Here's how the part is built. I have some questions about the finished solid (model axes, mm). A direction names the side the tool comes from. Give positions to 0.01 mm unless a question says otherwise; leave off trailing zeros. Loops run counter-clockwise (first coordinate to the right, second up) from the corner with the lowest first, then second, coordinate; pieces in that order, holes last. Notation, with made-up numbers: (24.25, 79) - (56.25, 79) arc R12 cw to (56.25, 98) - close; hole circle Ø2 at (12.5, 84.5). An arc over 180 degrees is marked (long way). Use a Markdown table: item, result.
Autodesk Inventor part; units mm, degrees
ref_plane "r_pin_XY" through (0, 0, 0) normal (0, 1, 0) x (1, 0, 0)
ref_plane "r_pin_YZ" through (0, 0, 0) normal (1, 0, 0) x (0, 0, -1)
ref_plane "r_pin_ZX" through (0, 0, 0) normal (0, 0, -1) x (0, 1, 0)
sketch "Sketch_1" plane through (0, 0, 0) normal (0, 0, 1) x (1, 0, 0)
  line L0 (0, -20.5) -> (0, 20.5)
  line L1 (0, 20.5) -> (4.6, 20.5)
  line L2 (4.6, 20.5) -> (4.6, -20.5)
  line L3 (4.6, -20.5) -> (0, -20.5)
  line L4 (0, -20.5) -> (0, 20.5)
revolve "Revolution1" add sketch "Sketch_1" angle 360 about axis through (0, -20.5, 0) along (0, -1, 0)
sketch "Sketch_2" plane through (0, 0, -4.6) normal (0, 0, 1) x (1, 0, 0)
  line L0 (0, 20.5) -> (0, -20.5)
  line L1 (0, -20.5) -> (10.5, -20.5)
  arc A0 (10.5, -20.5) -> (18, -13) centre (10.5, -13) ccw
  line L2 (18, -13) -> (18, 13)
  arc A1 (18, 13) -> (10.5, 20.5) centre (10.5, 13) ccw
  line L3 (10.5, 20.5) -> (0, 20.5)
extrude "Extrusion1" add sketch "Sketch_2" along normal blind 2
sketch "Sketch_3" plane through (0, 0, 0) normal (0, 0, 1) x (1, 0, 0)
  line L0 (-41, 41) -> (-41, -41)
  line L1 (-41, -41) -> (41, -41)
  line L2 (41, -41) -> (41, 41)
  line L3 (41, 41) -> (-41, 41)
  line L4 (-4.6, 20.5) -> (-4.6, 10.35)
  line L5 (-4.6, 10.35) -> (4.85, 10.35)
  line L6 (4.85, 10.35) -> (4.85, -0.2)
  line L7 (4.85, -0.2) -> (-4.6, -0.2)
  line L8 (-4.6, -0.2) -> (-4.6, -10.05)
  line L9 (-4.6, -10.05) -> (4.85, -10.05)
  line L10 (4.85, -10.05) -> (4.85, -20.5)
  line L11 (4.85, -20.5) -> (18, -20.5)
  line L12 (18, -20.5) -> (18, 20.5)
  line L13 (18, 20.5) -> (-4.6, 20.5)
extrude "Extrusion2" cut sketch "Sketch_3" along normal mid plane 82
sketch "Sketch_4" plane through (0, 0, 0) normal (0, 0, 1) x (1, 0, 0)
  line L0 (0, -20.5) -> (0, 20.5)
  line L1 (0, 20.5) -> (2.5, 20.5)
  line L2 (2.5, 20.5) -> (2.5, -20.5)
  line L3 (2.5, -20.5) -> (0, -20.5)
  line L4 (0, -20.5) -> (0, 20.5)
revolve "Revolution2" cut sketch "Sketch_4" angle 360 about axis through (0, -20.5, 0) along (0, -1, 0)
sketch "Sketch_5" plane through (0, 12.5, 0) normal (0, 1, 0) x (1, 0, 0)
  line L0 (10.5, 2.6) -> (10.5, 4.6)
  line L1 (10.5, 4.6) -> (13.25, 4.6)
  line L2 (13.25, 4.6) -> (13.25, 2.6)
  line L3 (13.25, 2.6) -> (10.5, 2.6)
  line L4 (10.5, 2.6) -> (10.5, 4.6)
revolve "Revolution3" cut sketch "Sketch_5" angle 360 about axis through (10.5, 12.5, -2.6) along (0, 0, 1)
sketch "Sketch_7" plane through (0, -12.5, 0) normal (0, 1, 0) x (1, 0, 0)
  line L0 (10.5, 2.6) -> (10.5, 4.6)
  line L1 (10.5, 4.6) -> (13.25, 4.6)
  line L2 (13.25, 4.6) -> (13.25, 2.6)
  line L3 (13.25, 2.6) -> (10.5, 2.6)
  line L4 (10.5, 2.6) -> (10.5, 4.6)
revolve "Revolution4" cut sketch "Sketch_7" angle 360 about axis through (10.5, -12.5, -2.6) along (0, 0, 1)
ref_plane "r_pin_XY" through (0, 0, 0) normal (0, 1, 0) x (1, 0, 0)
ref_plane "r_pin_YZ" through (0, 0, 0) normal (1, 0, 0) x (0, 0, -1)
ref_plane "r_pin_ZX" through (0, 0, 0) normal (0, 0, -1) x (0, 1, 0)
ref_plane "hole1r_to_bolt_XY" through (10.5, 12.5, -2.6) normal (0, 0, 1) x (1, 0, 0)
ref_plane "hole1r_to_bolt_YZ" through (10.5, 12.5, -2.6) normal (1, 0, 0) x (0, 1, 0)
ref_plane "hole1r_to_bolt_ZX" through (10.5, 12.5, -2.6) normal (0, 1, 0) x (0, 0, 1)
ref_plane "hole2r_to_bolt_XY" through (10.5, -12.5, -2.6) normal (0, 0, 1) x (1, 0, 0)
ref_plane "hole2r_to_bolt_YZ" through (10.5, -12.5, -2.6) normal (1, 0, 0) x (0, 1, 0)
ref_plane "hole2r_to_bolt_ZX" through (10.5, -12.5, -2.6) normal (0, 1, 0) x (0, 0, 1)
ref_plane "hole3r_to_bolt_XY" through (10.5, 0, -2.6) normal (0, 0, 1) x (1, 0, 0)
ref_plane "hole3r_to_bolt_YZ" through (10.5, 0, -2.6) normal (1, 0, 0) x (0, 1, 0)
ref_plane "hole3r_to_bolt_ZX" through (10.5, 0, -2.6) normal (0, 1, 0) x (0, 0, 1)
properties part number "SHHPS5-2-pin"
(1) Suppose I cut it at B-B on y = -12.5. Write out the boundary of the cut face in (x, z), plus the area to 3 significant figures.
A:
| item | result |
|---|---|
| outline | (4.85, -4.6) - (7.75, -4.6) - (7.75, -2.6) - (4.85, -2.6) - close; (13.25, -4.6) - (18, -4.6) - (18, -2.6) - (13.25, -2.6) - close |
| area | 15.3 mm2 |
(2) If I drill on line 1 (Y direction, x = 10.5, z = -3.4); line 2 (Y direction, x = -1.5, z = 3); line 3 (Z direction, x = 0, y = 15), over which ranges is the centre line in solid material (lowest first)?
A:
| item | result |
|---|---|
| line 1 | -20.5 to -15.25, -9.75 to 9.75, 15.25 to 20.5 |
| line 2 | -10.05 to -0.2, 10.35 to 20.5 |
| line 3 | -4.6 to -2.5, 2.5 to 4.6 |
(3) We'd pull the mould along X, two halves only. Please class faces 4 (the face through (13.12, 13.33, -3.59)), 5 (the face through (2, -0.2, -2)), 6 (the face through (4.85, -15, -4)): pulls with the +X half, pulls with the -X half, needs draft (parallel to the pull), parting line crosses it, or undercut.
A:
| item | result |
|---|---|
| face 4 | undercut |
| face 5 | needs draft |
| face 6 | pulls with the -X half |
(4) Suppose I cut it at C-C on z = 0. Write out the boundary of the cut face in (x, y), plus the area to 3 significant figures.
A:
| item | result |
|---|---|
| outline | (-4.6, -10.05) - (-2.5, -10.05) - (-2.5, -0.2) - (-4.6, -0.2) - close; (-4.6, 10.35) - (-2.5, 10.35) - (-2.5, 20.5) - (-4.6, 20.5) - close; (2.5, -10.05) - (4.6, -10.05) - (4.6, -0.2) - (2.5, -0.2) - close; (2.5, 10.35) - (4.6, 10.35) - (4.6, 20.5) - (2.5, 20.5) - close |
| area | 84.0 mm2 |
(5) Suppose I cut it at A-A on y = 12.5. Write out the boundary of the cut face in (x, z), plus the area to 3 significant figures.
A:
| item | result |
|---|---|
| outline | (0, -4.6) - (7.75, -4.6) - (7.75, -2.6) - (3.79, -2.6) arc R4.6 ccw (long way) to start; (13.25, -4.6) - (18, -4.6) - (18, -2.6) - (13.25, -2.6) - close; hole circle Ø5 at (0, 0) |
| area | 66.5 mm2 |
(6) Will these pins go through, and if not, where does the flat tip stop? pin 1 (1 mm diameter, centred on x = -1.5, y = -5, fed in from +Z); pin 2 (3 mm diameter, centred on x = 2, z = 1, fed in from -Y); pin 3 (3.5 mm diameter, centred on x = 10.5, y = -12.5, fed in from +Z); pin 4 (1 mm diameter, centred on y = 6, z = -3.5, fed in from -X).
A:
| item | result |
|---|---|
| pin 1 | z = 4.49 |
| pin 2 | y = -10.05 |
| pin 3 | through |
| pin 4 | x = 4.85 |
(7) Suppose I cut it at D-D on y = -2. Write out the boundary of the cut face in (x, z), plus the area to 3 significant figures.
A:
| item | result |
|---|---|
| outline | (0, -4.6) - (18, -4.6) - (18, -2.6) - (3.79, -2.6) arc R4.6 ccw (long way) to start; hole circle Ø5 at (0, 0) |
| area | 77.5 mm2 |
(8) On a 3-axis mill with a long thin cutter (end or side, diameter ignored), from which of +Z, -Z, +X, -X, +Y, -Y can I reach the whole of each face in a straight line? I mean faces 1 (the face through (9, 0, -4.6)), 2 (the face through (4.85, 5, -4)), 3 (the face through (2, -10.05, -2)). Say none if no direction works.
A:
| item | result |
|---|---|
| face 1 | -Z, +X, -X, +Y, -Y |
| face 2 | +Z, -Z, -X |
| face 3 | +Z, -Z, -X, -Y |
